Job drawing, mm, ordinate dimensions from the low corner. One solid piece. Round coordinates to 2 decimals unless told otherwise and drop trailing zeros. Write each loop counter-clockwise with the first axis right and the second up, starting at its lowest first coordinate (ties: lowest second). Pieces come first, ordered by that corner, then holes.
1) Saw through at D-D on x = 43.82. Write the cut outline in (y, z) (3 decimals), and give its area (3 significant figures).
2) Saw through at B-B on x = 33.82. Write the cut outline in (y, z) (3 decimals).
3) Drill centre lines: L1, parallel to X at y = 4.65, z = 25; L2, parallel to X at y = 2.05, z = 21; L3, parallel to X at y = 2.5, z = 55.25. Where is each one in solid material? Low to high.
4) Saw through at C-C on z = 9.6. Write the cut outline in (x, y).
5) Saw through at A-A on z = 24.75. Write the cut outline in (x, y), and give its area (3 significant figures).
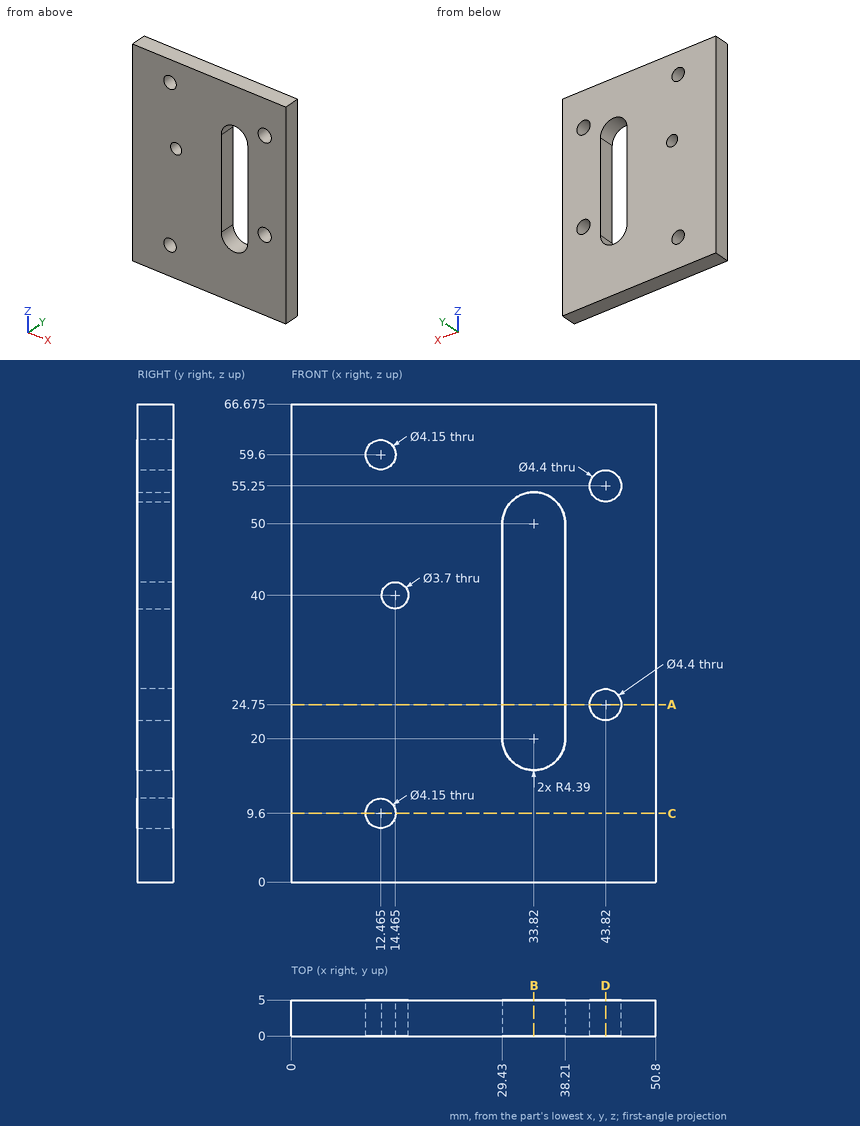
Completed:
1. outline: (0, 0) - (5, 0) - (5, 22.55) - (0, 22.55) - close; (0, 26.95) - (5, 26.95) - (5, 53.05) - (0, 53.05) - close; (0, 57.45) - (5, 57.45) - (5, 66.675) - (0, 66.675) - close
1. area: 289 mm2
2. outline: (0, 0) - (5, 0) - (5, 15.61) - (0, 15.61) - close; (0, 54.39) - (5, 54.39) - (5, 66.675) - (0, 66.675) - close
3. L1: x = 0 to 29.43, 38.21 to 41.63, 46.01 to 50.8
3. L2: x = 0 to 29.43, 38.21 to 50.8
3. L3: x = 0 to 41.62, 46.02 to 50.8
4. outline: (0, 0) - (10.39, 0) - (10.39, 5) - (0, 5) - close; (14.54, 0) - (50.8, 0) - (50.8, 5) - (14.54, 5) - close
5. outline: (0, 0) - (29.43, 0) - (29.43, 5) - (0, 5) - close; (38.21, 0) - (41.62, 0) - (41.62, 5) - (38.21, 5) - close; (46.02, 0) - (50.8, 0) - (50.8, 5) - (46.02, 5) - close
5. area: 188 mm2
